Source: CAD feature listing. Evaluate the final solid. Frame: model axes, mm. A direction names the side the tool comes from. Coordinates: 2 decimals unless noted, no trailing zeros. Loops run counter-clockwise (first coordinate to the right, second up) from the corner with the lowest first, then second, coordinate; pieces in that order, holes last. Notation, with made-up numbers: M 72,-19 L 112,-19 A17 cw 112,-10 Z; hole C -31.75,59 d6. An arc over 180 degrees is marked long. Write each question's results on one line, items separated by ' | '. Start each with the question number.
Autodesk Inventor part; units mm, degrees
ref_plane "YZ Plane" through (0, 0, 0) normal (1, 0, 0) x (0, 1, 0)
ref_plane "XZ Plane" through (0, 0, 0) normal (0, 1, 0) x (-1, 0, 0)
ref_plane "XY Plane" through (0, 0, 0) normal (0, 0, 1) x (1, 0, 0)
sketch "Sketch1" plane through (0, 0, 0) normal (0, 1, 0) x (-1, 0, 0)
  line L0 (0, 0) -> (80, 0)
  line L1 (80, 0) -> (80, -80)
  line L2 (80, -80) -> (0, -80)
  line L3 (0, -80) -> (0, 0)
  dimension "d0" = 80
  dimension "d1" = 80
extrude "Extrusion1" add sketch "Sketch1" along normal blind 30
sketch "Sketch2" plane through (0, 30, 0) normal (0, 1, 0) x (1, 0, 0)
  line L0 (-85, -5) -> (5, -5)
  line L1 (5, -5) -> (5, 85)
  line L2 (5, 85) -> (-85, 85)
  line L3 (-85, 85) -> (-85, -5)
  line L4 (-80, 80) -> (-80, 0)
  line L5 (0, 80) -> (-80, 80)
  line L6 (-80, 0) -> (0, 0)
  line L7 (0, 0) -> (0, 80)
  dimension "d4" = 5
  dimension "d5" = 5
  dimension "d6" = 5
  dimension "d7" = 5
extrude "Extrusion2" add sketch "Sketch2" along normal blind 45 contours L3 L2 L1 L0 | L5 L7 L6 L4
sketch "Sketch3" plane through (0, 75, 0) normal (0, 1, 0) x (1, 0, 0)
  line L0 (0, 0) -> (-80, 0)
  line L1 (-80, 0) -> (-80, 80)
  line L2 (-80, 80) -> (0, 80)
  line L3 (0, 80) -> (0, 0)
  line L4 (-85, 85) -> (-85, -5)
  line L5 (5, 85) -> (-85, 85)
  dimension "d10" = 5
  dimension "d11" = 5
extrude "Extrusion3" cut sketch "Sketch3" against normal blind 40
sketch "Sketch4" plane through (0, 35, 0) normal (0, 1, 0) x (1, 0, 0)
  line L0 (-75, 5) -> (-5, 5)
  line L1 (-5, 5) -> (-5, 75)
  line L2 (-5, 75) -> (-75, 75)
  line L3 (-75, 75) -> (-75, 5)
  line L4 (-80, 80) -> (0, 80)
  line L5 (0, 80) -> (0, 0)
  line L6 (0, 0) -> (-80, 0)
  line L7 (-80, 0) -> (-80, 80)
  dimension "d14" = 5
  dimension "d15" = 5
  dimension "d16" = 5
  dimension "d17" = 5
extrude "Extrusion4" cut sketch "Sketch4" against normal blind 30 contours L3 L2 L1 L0
sketch "Sketch5" plane through (5, 30, 5) normal (1, 0, 0) x (0, 0, -1)
  circle A0 centre (65, 32.5) radius 2.75
  line L0 (0, 45) -> (90, 45)
  line L1 (90, 0) -> (90, 45)
  point P0 (5, -30)
  dimension "d20" = 5.5
  dimension "d21" = 12.5
  dimension "d22" = 25
extrude "Extrusion5" cut sketch "Sketch5" against normal through all
sketch "Sketch6" plane through (5, 30, 5) normal (1, 0, 0) x (0, 0, -1)
  line L0 (75.5, 35) -> (80, 35)
  line L1 (80, 35) -> (80, 25.5)
  line L2 (80, 25.5) -> (75.5, 25.5)
  line L3 (75.5, 25.5) -> (75.5, 35)
  line L4 (90, 0) -> (90, 45)
  line L5 (0, 45) -> (90, 45)
  point P0 (5, -30)
  dimension "d25" = 10
  dimension "d26" = 4.5
  dimension "d27" = 9.5
  dimension "d28" = 10
extrude "Extrusion6" cut sketch "Sketch6" against normal blind 10
chamfer "Chamfer1" distance 2 angle 45 4 edges at (5, 60.25, -70.5) (5, 65, -72.75) (5, 60.25, -75) (5, 55.5, -72.75)
sketch "Sketch8" plane through (-85, 30, -85) normal (-1, 0, 0) x (0, 0, 1)
  line L0 (23, 25) -> (27.5, 25)
  line L1 (27.5, 25) -> (27.5, 15.5)
  line L2 (27.5, 15.5) -> (23, 15.5)
  line L3 (23, 15.5) -> (23, 25)
  line L4 (13.5, 25) -> (18, 25)
  line L5 (18, 25) -> (18, 15.5)
  line L6 (18, 15.5) -> (13.5, 15.5)
  line L7 (13.5, 15.5) -> (13.5, 25)
  line L8 (32.5, 25) -> (37, 25)
  line L9 (37, 25) -> (37, 15.5)
  line L10 (37, 15.5) -> (32.5, 15.5)
  line L11 (32.5, 15.5) -> (32.5, 25)
  line L12 (0, 45) -> (90, 45)
  line L13 (0, 0) -> (0, 45)
  point P0 (85, -30)
  dimension "d39" = 4.5
  dimension "d40" = 9.5
  dimension "d41" = 4.5
  dimension "d42" = 4.5
  dimension "d43" = 20
  dimension "d44" = 23
  dimension "d45" = 5
  dimension "d46" = 5
extrude "Extrusion7" cut sketch "Sketch8" against normal blind 10
chamfer "Chamfer2" distance 2 angle 45 12 edges at (-85, 55, -69.25) (-85, 50.25, -71.5) (-85, 50.25, -67) (-85, 45.5, -69.25) (-85, 50.25, -62) (-85, 55, -59.75) (-85, 50.25, -57.5) (-85, 45.5, -59.75) (-85, 50.25, -52.5) (-85, 55, -50.25) (-85, 50.25, -48) (-85, 45.5, -50.25)
properties part number "BlackBoxBottomFall2019"
Item 1: Cut plane B-B (z = -60). Count the separate pieces of the cut face and the enclosed holes in it, then the cut area to 3 significant figures.
Item 2: First-contact query: pin 1 Ø12 at (y, z) = (15, -34.5) entering from -X; pin 2 Ø5 at (y, z) = (62.5, -60) entering from +X; pin 3 Ø3.5 at (x, z) = (-82, -60.5) entering from -Y; pin 4 Ø5 at (x, z) = (-51.5, -56.5) entering from +Y. Flat tips, straight axial feed; report the tip coordinate or a pass-through.
Item 3: Line query: probe 1 along Y at (x, z) = (-83, -60); probe 2 along X at (y, z) = (34.5, -13); probe 3 along X at (y, z) = (10, -7.5). Output: solid intervals per line, ascending.
Item 4: Cut plane A-A (y = 62.5). Output: boundary loops of the cut face in (x, z), then the cut area to 3 significant figures.
Item 5: Access query for faces 1 (the flat face through (-40, 20, -5)), 2 (the flat face through (-85, 52, -41)), 3 (the flat face through (-80, 15, -39)), 4 (the flat face through (-82, 45.5, -69)), 5 (the flat face through (2, 60, -75)). Directions: +Z, -Z, +X, -X, +Y, -Y. A direction counts if a zero-diameter tool reaches every point of the face in a straight line with its end or side. Return the directions, or none.
Item 6: Mould query, pull axis X, two halves, no side actions, for faces 6 (the flat face through (-5, 20, -40)), 7 (the flat face through (2, 65, -73)), 8 (the flat face through (0, 15, -41)). Classes: +X half, -X half, draft (parallel to the pull), parting line (faces both ways), or undercut.
Item 7: Cut plane C-C (x = -3.5). Output: boundary loops of the cut face in (y, z).
Item 8: Cut plane D-D (z = -7). Output: boundary loops of the cut face in (x, y), then the cut area to 3 significant figures.
Response values:
1) separate pieces: 4 | enclosed holes: 0 | area: 1,040 mm2
2) pin 1: stops at x = -80 | pin 2: passes through | pin 3: stops at y = 30 | pin 4: stops at y = 5
3) probe 1: y = 30 to 45.5, 55 to 59.75, 65.25 to 75 | probe 2: x = -85 to -75, -5 to 5 | probe 3: x = -80 to -75, -5 to 0
4) outline: M -85,-85 L 5,-85 L 5,-77 L 3,-75 L 0,-75 L 0,-80 L -80,-80 L -80,-62.75 L -85,-62.75 Z; M -85,-57.25 L -80,-57.25 L -80,0 L 0,0 L 0,-57.25 L 5,-57.25 L 5,5 L -85,5 Z; M 0,-70.5 L 3,-70.5 L 5,-68.5 L 5,-62.75 L 0,-62.75 Z | area: 1,620 mm2
5) face 1: +Y | face 2: +Z, -Z, -X, +Y, -Y | face 3: +Z, -Z, -X, -Y | face 4: -X | face 5: +X
6) face 6: undercut | face 7: draft | face 8: +X half
7) outline: M 0,-80 L 30,-80 L 30,-85 L 75,-85 L 75,-80 L 35,-80 L 35,0 L 75,0 L 75,5 L 30,5 L 30,0 L 0,0 Z
8) outline: M -85,30 L -80,30 L -80,0 L 0,0 L 0,30 L 5,30 L 5,75 L 0,75 L 0,35 L -5,35 L -5,5 L -75,5 L -75,35 L -80,35 L -80,75 L -85,75 Z | area: 1,150 mm2
